Input: part model. Units: mm. Frame: model coordinates. Face numbers are marked on the shaded views. A direction names the side the tool comes from. Round coordinates to 2 decimals unless told otherwise and drop trailing zeros. Order: outer loops, then holes, each group sorted by start corner. A loop starts at its lowest first (then second) coordinate and runs counter-clockwise, first axis right, second up.
Item 1: Cut plane B-B on x = 0. Output: boundary loops of the cut face in (y, z).
Item 2: Reachability of the marked faces 1 and 2 from +Z, -Z, +X, -X, +Y, -Y: full face, straight path, thin tool, end or side. Return the list, or none.
Item 3: Line query: L1, parallel to Y at x = -7, z = -5.75; L2, parallel to Y at x = -4, z = -5.75; L3, parallel to Z at x = -8.75, y = 89.5. Output: solid intervals per line, ascending.
Item 4: Cut plane A-A on z = 0. Output: boundary loops of the cut face in (x, y).
Item 5: Cut plane D-D on y = 26.5. Output: boundary loops of the cut face in (x, z), then the cut area to 3 significant figures.
Item 6: Cut plane C-C on y = 12. Output: boundary loops of the cut face in (x, z), then the cut area to 3 significant figures.
Item 7: First-contact query: pin 1 (4 mm diameter, centred on x = -10.5, y = 99, fed in from -Z); pin 2 (4 mm diameter, centred on x = 2, y = 76.5, fed in from -Z); pin 3 (2 mm diameter, centred on y = 73, z = -5.5, fed in from -X). Flat tips, straight axial feed; report the tip coordinate or a pass-through.
Solid Edge part; units mm, degrees
sketch "Sketch1" plane through (0, 0, 0) normal (0, 0, 1) x (1, 0, 0)
  line L0 (11.9126, 97.2312) -> (11.9126, 28.194)
  line L1 (11.9126, 28.194) -> (9.017, 28.194)
  line L2 (9.017, 28.194) -> (9.017, 13.462)
  line L3 (9.017, 13.462) -> (6.2611, 13.462)
  line L4 (6.2611, 13.462) -> (6.2611, 0)
  line L5 (6.2611, 0) -> (0, 0)
  line L6 (0, 0) -> (0, 100.7312)
  line L7 (0, 100.7312) -> (12.5095, 100.7312)
  line L8 (12.5095, 100.7312) -> (12.5095, 97.2312)
  line L9 (12.5095, 97.2312) -> (11.9126, 97.2312)
revolve "RevolvedProtrusion1" add sketch "Sketch1" angle 360 about axis through (0, 0, 0) along (0, 1, 0)
sketch "Sketch2" plane through (0, 0, 0) normal (0, 0, 1) x (1, 0, 0)
  line L0 (7.8095, 97.2312) -> (12.5095, 97.2312)
  line L1 (12.5095, 97.2312) -> (12.5095, 100.7312)
  line L2 (12.5095, 100.7312) -> (10.7463, 100.7312)
  line L3 (10.7463, 100.7312) -> (7.8095, 97.2312)
extrude "Cutout1" cut sketch "Sketch2" along normal mid plane 9
mirror "Mirror1" about plane through (0, 0, 0) normal (1, 0, 0) of "Cutout1"
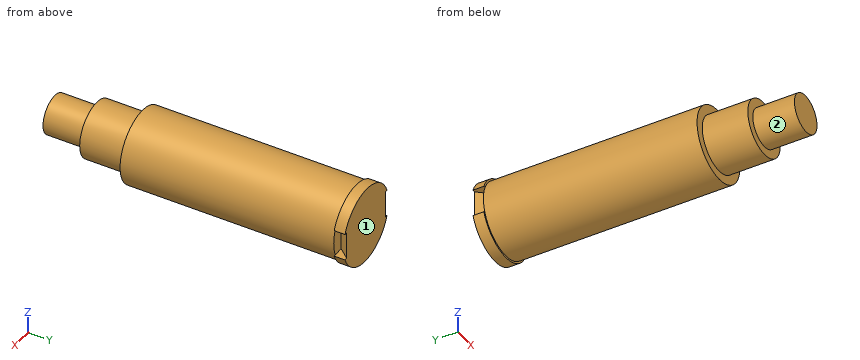
From the geometry:
1. outline: (0, -6.26) - (13.46, -6.26) - (13.46, -9.02) - (28.19, -9.02) - (28.19, -11.91) - (97.23, -11.91) - (97.23, -12.51) - (100.73, -12.51) - (100.73, 12.51) - (97.23, 12.51) - (97.23, 11.91) - (28.19, 11.91) - (28.19, 9.02) - (13.46, 9.02) - (13.46, 6.26) - (0, 6.26) - close
2. face 1: +Z, -Z, +X, -X, +Y
2. face 2: -Y
3. L1: y = 28.19 to 100.73
3. L2: y = 13.46 to 100.73
3. L3: z = -8.08 to 8.08
4. outline: (-11.91, 28.19) - (-9.02, 28.19) - (-9.02, 13.46) - (-6.26, 13.46) - (-6.26, 0) - (6.26, 0) - (6.26, 13.46) - (9.02, 13.46) - (9.02, 28.19) - (11.91, 28.19) - (11.91, 97.23) - (7.81, 97.23) - (10.75, 100.73) - (-10.75, 100.73) - (-7.81, 97.23) - (-11.91, 97.23) - close
5. outline: circle Ø18.03 at (0, 0)
5. area: 255 mm2
6. outline: circle Ø12.52 at (0, 0)
6. area: 123 mm2
7. pin 1: stops at z = -9.18
7. pin 2: stops at z = -11.91
7. pin 3: stops at x = -11.03
